For this review, take the finished solid that the model builds, in its own axes (mm). Face numbers are marked on the shaded views. A direction names the side the tool comes from. Round coordinates to 2 decimals unless told otherwise and drop trailing zeros. Order: outer loops, then holes, each group sorted by start corner. A loop starts at its lowest first (then second) coordinate and runs counter-clockwise, first axis right, second up. Notation, with made-up numbers: M -16,41.25 L 29,41.25 A24 ccw 29,75.25 Z; hole C 0.5,41 d11. An arc over 180 degrees is marked long. Write item = value, one per line. Start each with the question number.
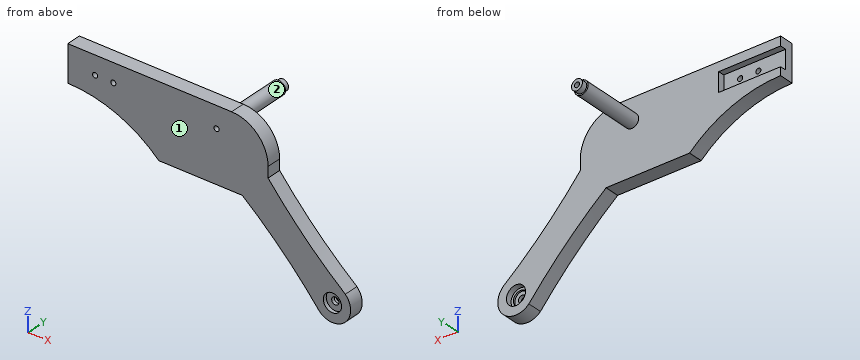
from build123d import *

# Parameters (mm, degrees)
BOSS_EXTRUDE1_DEPTH      = 8
CUT_EXTRUDE1_DEPTH       = 121.027140353
CUT_EXTRUDE1_DEPTH_BACK  = 121.027140353
SKETCH2_R                = 1.4
CUT_EXTRUDE2_DEPTH       = 121.027140353
SKETCH4_R                = 5.25
CUT_EXTRUDE3_DEPTH       = 3.2
SKETCH5_R                = 4
CUT_EXTRUDE4_DEPTH       = 1
SKETCH6_R                = 5
CUT_EXTRUDE5_DEPTH       = 2
CUT_EXTRUDE6_DEPTH       = 120.833861747
CUT_EXTRUDE6_DEPTH_BACK  = 120.833861747
SKETCH7_R                = 2
SKETCH9_R                = 3.75
BOSS_EXTRUDE2_DEPTH      = 35
SKETCH10_R               = 3
BOSS_EXTRUDE3_DEPTH      = 3
CUT_EXTRUDE8_DEPTH       = 129.29074176
CUT_EXTRUDE8_DEPTH_BACK  = 129.29074176
SKETCH11_R               = 1.4
CUT_EXTRUDE9_DEPTH       = 126.644396697
CUT_EXTRUDE9_DEPTH_BACK  = 126.644396697
SKETCH13_W               = 34
SKETCH13_H               = 10.5
CUT_EXTRUDE10_DEPTH      = 3.5
FILLET2_R                = 20
CUT_EXTRUDE11_DEPTH      = 127.746851721
CUT_EXTRUDE11_DEPTH_BACK = 127.746851721
SKETCH14_R               = 1.4


with BuildPart() as part:
    # Sketch1 → Boss-Extrude1 (new body)
    with BuildSketch(Plane(origin=(0, 0, 0), x_dir=(1, 0, 0), z_dir=(0, 1, 0))):
        with BuildLine():
            Line((40.857864376, 20), (83.284271247, 62.426406871))
            ThreePointArc((83.284271247, 62.426406871), (97.426406871, 62.426406871), (97.426406871, 48.284271247))
            Line((97.426406871, 48.284271247), (55, 5.857864376))
            Line((55, 5.857864376), (55, -20))
            Line((55, -20), (-55, -20))
            Line((-55, -20), (-55, 20))
            Line((-55, 20), (40.857864376, 20))
        make_face()
    extrude(amount=BOSS_EXTRUDE1_DEPTH)

    # Sketch2 → Cut-Extrude1 (cut, two sides: drawn at the far end of the back side and taken through both)
    with BuildSketch(Plane(origin=(0, 8, 0), x_dir=(1, 0, 0), z_dir=(0, 1, 0)).offset(-CUT_EXTRUDE1_DEPTH_BACK)):
        with Locations(Location((90.355339059, 55.355339059, 0), (0, 0, 270))):
            Circle(SKETCH2_R)
        with Locations(Location((26.715728753, -8.284271247, 0), (0, 0, 270))):
            Circle(SKETCH2_R)
    extrude(amount=CUT_EXTRUDE1_DEPTH + CUT_EXTRUDE1_DEPTH_BACK, mode=Mode.SUBTRACT)

    # Sketch3 → Cut-Extrude2 (cut, symmetric)
    with BuildSketch(Plane(origin=(0, 8, 0), x_dir=(1, 0, 0), z_dir=(0, 1, 0))):
        with BuildLine():
            Line((40.857864376, 20), (83.284271247, 62.426406871))
            ThreePointArc((83.284271247, 62.426406871), (63.134392976, 40.149878272), (40.857864376, 20))
        make_face()
    cut_extrude2 = extrude(amount=CUT_EXTRUDE2_DEPTH, both=True, mode=Mode.SUBTRACT)

    # Mirror1: Cut-Extrude2 across plane
    add(cut_extrude2.mirror(Plane(origin=(17.5, 0, 17.5), x_dir=(-0.7071067811865461, 0, 0.707106781186549), z_dir=(0.7071067811865492, 0, 0.7071067811865459))), mode=Mode.SUBTRACT)

    # Sketch4 → Cut-Extrude3 (cut)
    with BuildSketch(Plane(origin=(0, 8, 0), x_dir=(1, 0, 0), z_dir=(0, 1, 0))):
        with Locations(Location((90.355339059, 55.355339059, 0), (0, 0, 270))):
            Circle(SKETCH4_R)
    extrude(amount=-CUT_EXTRUDE3_DEPTH, mode=Mode.SUBTRACT)

    # Sketch5 → Cut-Extrude4 (cut)
    with BuildSketch(Plane(origin=(0, 4.8, 0), x_dir=(1, 0, 0), z_dir=(0, 1, 0))):
        with Locations(Location((90.355339059, 55.355339059, 0), (0, 0, 270))):
            Circle(SKETCH5_R)
    extrude(amount=-CUT_EXTRUDE4_DEPTH, mode=Mode.SUBTRACT)

    # Sketch6 → Cut-Extrude5 (cut)
    with BuildSketch(Plane.XZ):
        with Locations(Location((90.355339059, -55.355339059, 0), (0, 0, 270))):
            Circle(SKETCH6_R)
    extrude(amount=-CUT_EXTRUDE5_DEPTH, mode=Mode.SUBTRACT)

    # Sketch7 → Cut-Extrude6 (cut, two sides: drawn at the far end of the back side and taken through both)
    with BuildSketch(Plane(origin=(0, 3.8, 0), x_dir=(1, 0, 0), z_dir=(0, 1, 0)).offset(-CUT_EXTRUDE6_DEPTH_BACK)):
        with Locations(Location((90.355339059, 55.355339059, 0), (0, 0, 270))):
            Circle(SKETCH7_R)
    extrude(amount=CUT_EXTRUDE6_DEPTH + CUT_EXTRUDE6_DEPTH_BACK, mode=Mode.SUBTRACT)

    # Sketch9 → Boss-Extrude2 (add)
    with BuildSketch(Plane(origin=(0, 8, 0), x_dir=(1, 0, 0), z_dir=(0, 1, 0))):
        with Locations(Location((26.715728753, -8.284271247, 0), (0, 0, 270))):
            Circle(SKETCH9_R)
    extrude(amount=BOSS_EXTRUDE2_DEPTH)

    # Sketch10 → Boss-Extrude3 (add)
    with BuildSketch(Plane(origin=(0, 43, 0), x_dir=(1, 0, 0), z_dir=(0, 1, 0))):
        with Locations(Location((26.715728753, -8.284271247, 0), (0, 0, 270))):
            Circle(SKETCH10_R)
    extrude(amount=BOSS_EXTRUDE3_DEPTH)

    # Sketch11 → Cut-Extrude8 (cut, two sides: drawn at the far end of the back side and taken through both)
    with BuildSketch(Plane(origin=(0, 46, 0), x_dir=(1, 0, 0), z_dir=(0, 1, 0)).offset(-CUT_EXTRUDE8_DEPTH_BACK)):
        with Locations(Location((26.715728753, -8.284271247, 0), (0, 0, 270))):
            Circle(SKETCH11_R)
    extrude(amount=CUT_EXTRUDE8_DEPTH + CUT_EXTRUDE8_DEPTH_BACK, mode=Mode.SUBTRACT)

    # Sketch12 → Cut-Extrude9 (cut, two sides: drawn at the far end of the back side and taken through both)
    with BuildSketch(Plane(origin=(0, 8, 0), x_dir=(1, 0, 0), z_dir=(0, 1, 0)).offset(-CUT_EXTRUDE9_DEPTH_BACK)):
        with BuildLine():
            Line((-55, 0), (-55, 20))
            Line((-55, 20), (-5, 20))
            ThreePointArc((-5, 20), (-28.074175964, 5.185439911), (-55, 0))
        make_face()
    extrude(amount=CUT_EXTRUDE9_DEPTH + CUT_EXTRUDE9_DEPTH_BACK, mode=Mode.SUBTRACT)

    # Sketch13 → Cut-Extrude10 (cut)
    with BuildSketch(Plane(origin=(0, 8, 0), x_dir=(1, 0, 0), z_dir=(0, 1, 0))):
        with Locations((-38, -9.75)):
            Rectangle(SKETCH13_W, SKETCH13_H)
    extrude(amount=-CUT_EXTRUDE10_DEPTH, mode=Mode.SUBTRACT)

    # Fillet2
    fillet2_edges = [part.edges().sort_by_distance(p)[0] for p in [
        (55, 4, 20),
    ]]
    fillet(fillet2_edges, radius=FILLET2_R)

    # Sketch14 → Cut-Extrude11 (cut, two sides: drawn at the far end of the back side and taken through both)
    with BuildSketch(Plane(origin=(0, 4.5, 0), x_dir=(1, 0, 0), z_dir=(0, 1, 0)).offset(-CUT_EXTRUDE11_DEPTH_BACK)):
        with Locations(Location((-40, -9.75, 0), (0, 0, 270))):
            Circle(SKETCH14_R)
        with Locations(Location((-30, -9.75, 0), (0, 0, 270))):
            Circle(SKETCH14_R)
    extrude(amount=CUT_EXTRUDE11_DEPTH + CUT_EXTRUDE11_DEPTH_BACK, mode=Mode.SUBTRACT)


solid = part.part
(1) We need section A-A, the plane y = 28. Write out the cut boundary in (x, z).
(2) For line 1 along Z through (x, y) = (26.5, 39); line 2 along Z through (x, y) = (14, 2.5); line 3 along X through (y, z) = (2, 9), list the stretches that pass through material, from the lowest coordinate up.
(3) Insertion check: pin 1 (6 mm diameter, centred on x = 2.5, y = 7, fed in from -Z); pin 2 (6.5 mm diameter, centred on x = 90.36, z = -55.36, fed in from +Y); pin 3 (4.5 mm diameter, centred on y = 4.5, z = -1.5, fed in from +X); pin 4 (5 mm diameter, centred on y = 12.5, z = -6.5, fed in from +X). Each pin has a flat end and moves straight along its axis. Give the tip position at first contact, or say it passes through.
(4) We need section C-C, the plane x = -17.5. Write out the cut boundary in (y, z).
(5) We need section B-B, the plane x = 64. Write out the cut boundary in (y, z) (3 decimals).
(6) For the marked faces 1 and 2, list the 3-axis set-ups (+Z, -Z, +X, -X, +Y, -Y) from which the entire face can be reached by the end or side of a thin tool; tool diameter is ignored.
Values:
q1.outline = C 26.72,8.28 d7.5; hole C 26.72,8.28 d2.8
q2.line_1 = 4.54 to 6.9, 9.67 to 12.03
q2.line_2 = -20 to 20
q2.line_3 = -55 to -41.18, -38.82 to -31.18, -28.82 to 25.51, 27.92 to 52.86
q3.pin_1 = -20
q3.pin_2 = 3.8
q3.pin_3 = 55
q3.pin_4 = through
q4.outline = M 0,-10.45 L 8,-10.45 L 8,20 L 0,20 Z
q5.outline = M 0,-41.019 L 8,-41.019 L 8,-16.365 L 0,-16.365 Z
q6.face_1 = +Z, -Z, +X, -X, -Y
q6.face_2 = +Y
